Part model, mm, in its own coordinate system. Give positions to 0.01 mm unless a question says otherwise; leave off trailing zeros. Write each loop counter-clockwise with the first axis right and the second up, starting at its lowest first coordinate (ties: lowest second). Pieces come first, ordered by that corner, then holes. Notation, with made-up numbers: M 49,54 L 96,54 A16 cw 96,80 Z; hole C 22.5,8.5 d2. An arc over 180 degrees is marked long. Use a Markdown table: item, result.
```python
from build123d import *

# Parameters (mm, degrees)
SKETCH3_W                      = 333.036830712
SKETCH3_H                      = 85
BASE_FLANGE1_DEPTH             = 3
EDGE_FLANGE1_STRIP_W           = 13.4732
EDGE_FLANGE1_STRIP_H           = 3
EDGE_FLANGE1_STRIP_CUT_DEPTH   = 333.036830711
EDGE_FLANGE1_STRIP_2_W         = 13.4732
EDGE_FLANGE1_STRIP_2_H         = 3
EDGE_FLANGE1_STRIP_CUT_2_DEPTH = 333.036830711
EDGE_FLANGE1_DEPTH             = 333.036830711
EDGE_FLANGE1_BEND_DEPTH        = 333.036830711
SKETCH14_R                     = 4.1
CUT_EXTRUDE1_DEPTH             = 10
LPATTERN1_COUNT                = 3
LPATTERN1_PITCH                = 20
INDENT1_START                  = 23
INDENT1_DEPTH                  = 87
INDENT1_START_2                = 1066.181520764
INDENT1_2_DEPTH                = 11.708931468
INDENT1_START_3                = 23.50429019
INDENT1_3_DEPTH                = 85
INDENT1_START_4                = 1388.984464138
INDENT1_4_DEPTH                = 10.233887338
INDENT1_5_DEPTH                = 85
CUT_EXTRUDE2_DEPTH             = 10
LPATTERN2_COUNT                = 2
LPATTERN2_PITCH                = 101
LPATTERN2_COPY_1_SKETCH_R      = 4.1
LPATTERN2_COPY_1_DEPTH         = 10
LPATTERN2_COPY_2_SKETCH_R      = 4.1
LPATTERN2_COPY_2_DEPTH         = 10


with BuildPart() as part:
    # Base-Flange1: sheet metal written as solids
    # Sketch3 → Base-Flange1 (new body)
    with BuildSketch(Plane(origin=(-0.035963347, 187.801831242, 0), x_dir=(0.9999999816645936, 0.0001914962472965804, 0), z_dir=(-0.0001914962472965804, 0.9999999816645936, 0))):
        with Locations((1232.69993612, -66.00429019)):
            Rectangle(SKETCH3_W, SKETCH3_H)
    extrude(amount=-BASE_FLANGE1_DEPTH)

    # Edge-Flange1: sheet metal written as solids
    # Edge-Flange1 strip (on a plane across the edge) → Edge-Flange1 strip cut (cut)
    with BuildSketch(Plane(origin=(1399.182936963, 185.06977636, 108.50429019), x_dir=(0, 0, -1), z_dir=(-0.9999999816645935, -0.00019149624729661617, 0))):
        with Locations((-3, -1.5)):
            Rectangle(EDGE_FLANGE1_STRIP_W, EDGE_FLANGE1_STRIP_H)
    extrude(amount=EDGE_FLANGE1_STRIP_CUT_DEPTH, mode=Mode.SUBTRACT)

    # Edge-Flange1 strip 2 (on a plane across the edge) → Edge-Flange1 strip cut 2 (cut)
    with BuildSketch(Plane(origin=(1066.146112358, 185.006001057, 23.50429019), x_dir=(0, 0, 1), z_dir=(0.9999999816645935, 0.00019149624729661617, 0))):
        with Locations((-3, -1.5)):
            Rectangle(EDGE_FLANGE1_STRIP_2_W, EDGE_FLANGE1_STRIP_2_H)
    extrude(amount=EDGE_FLANGE1_STRIP_CUT_2_DEPTH, mode=Mode.SUBTRACT)

    # Edge-Flange1 section (on a plane across the edge) → Edge-Flange1 (add)
    with BuildSketch(Plane(origin=(1399.182936963, 185.06977636, 108.50429019), x_dir=(0, 0, -1), z_dir=(-0.9999999816645935, -0.00019149624729661617, 0))):
        with BuildLine():
            Line((0, 0.7366), (0, 12))
            Line((0, 12), (3, 12))
            Line((3, 12), (3, 0.7366))
            ThreePointArc((3, 0.7366), (3.215745145, 0.215745145), (3.7366, 0))
            Line((3.7366, 0), (3.7366, -3))
            ThreePointArc((3.7366, -3), (1.094424801, -1.905575199), (0, 0.7366))
        make_face()
    extrude(amount=EDGE_FLANGE1_DEPTH)

    # Edge-Flange1 section 2 (on a plane across the edge) → Edge-Flange1 bend (add)
    with BuildSketch(Plane(origin=(1066.146112358, 185.006001057, 23.50429019), x_dir=(0, 0, 1), z_dir=(0.9999999816645935, 0.00019149624729661617, 0))):
        with BuildLine():
            Line((0, 0.7366), (0, 12))
            Line((0, 12), (3, 12))
            Line((3, 12), (3, 0.7366))
            ThreePointArc((3, 0.7366), (3.215745145, 0.215745145), (3.7366, 0))
            Line((3.7366, 0), (3.7366, -3))
            ThreePointArc((3.7366, -3), (1.094424801, -1.905575199), (0, 0.7366))
        make_face()
    extrude(amount=EDGE_FLANGE1_BEND_DEPTH)

    # Sketch14 → Cut-Extrude1 (cut)
    with BuildSketch(Plane(origin=(-0.035963347, 187.801831242, 0), x_dir=(0.9999999816645936, 0.00019149624729658044, 0), z_dir=(-0.00019149624729658044, 0.9999999816645936, 0))):
        with Locations(Location((1152.844912527, -41.50429019, 0), (0, 0, 180))):
            Circle(SKETCH14_R)
        with Locations(Location((1213.814912527, -41.50429019, 0), (0, 0, 180))):
            Circle(SKETCH14_R)
        with Locations(Location((1152.844912527, -90.50429019, 0), (0, 0, 180))):
            Circle(SKETCH14_R)
        with Locations(Location((1213.814912527, -90.50429019, 0), (0, 0, 180))):
            Circle(SKETCH14_R)
    cut_extrude1 = extrude(amount=-CUT_EXTRUDE1_DEPTH, mode=Mode.SUBTRACT)

    # LPattern1: Cut-Extrude1 ×3
    with Locations(*[Vector(-0.9999999816645936, -0.00019149624729658041, 0) * (i * LPATTERN1_PITCH) for i in range(1, LPATTERN1_COUNT)]):
        add(cut_extrude1, mode=Mode.SUBTRACT)

    # Indent1: read off the stored shape, not the designer's step
    # Indent1 outline → Indent1 (cut)
    with BuildSketch(Plane.XY.offset(INDENT1_START)):
        with BuildLine():
            Line((1391.658769663, 190), (1390.104573792, 188.068047026))
            ThreePointArc((1390.104573792, 188.068047026), (1387.312839815, 180.67842019), (1389.429552771, 173.067908404))
            Line((1389.429552771, 173.067908404), (1390.14074534, 172))
            Line((1390.14074534, 172), (1399.185439777, 172))
            Line((1399.185439777, 172), (1401, 172))
            Line((1401, 172), (1401, 190))
            Line((1401, 190), (1391.658769663, 190))
        make_face()
        with BuildLine():
            Line((1076.353702039, 188.007964899), (1074.752112936, 190))
            Line((1074.752112936, 190), (1065, 190))
            Line((1065, 190), (1065, 172))
            Line((1065, 172), (1066.14860296, 172))
            Line((1066.14860296, 172), (1076.353013915, 172))
            Line((1076.353013915, 172), (1077.024720786, 173.00808405))
            ThreePointArc((1077.024720786, 173.00808405), (1079.143304168, 180.617808163), (1076.353702039, 188.007964899))
        make_face()
    extrude(amount=INDENT1_DEPTH, mode=Mode.SUBTRACT)

    # Sketch15 → Cut-Extrude2 (cut)
    with BuildSketch(Plane(origin=(-0.035963347, 187.801831242, 0), x_dir=(0.9999999816645936, 0.0001914962472966162, 0), z_dir=(-0.0001914962472966162, 0.9999999816645936, 0))):
        with BuildLine():
            Line((1290.140555319, -48.00429019), (1340.140555319, -48.00429019))
            ThreePointArc((1340.140555319, -48.00429019), (1358.140555319, -66.00429019), (1340.140555319, -84.00429019))
            Line((1340.140555319, -84.00429019), (1290.140555319, -84.00429019))
            ThreePointArc((1290.140555319, -84.00429019), (1272.140555319, -66.00429019), (1290.140555319, -48.00429019))
        make_face()
    extrude(amount=-CUT_EXTRUDE2_DEPTH, mode=Mode.SUBTRACT)

    # LPattern2: Cut-Extrude1 ×2
    with Locations(*[Vector(0.9999999816645935, 0.0001914962472965804, 0) * (i * LPATTERN2_PITCH) for i in range(1, LPATTERN2_COUNT)]):
        add(cut_extrude1, mode=Mode.SUBTRACT)

    # LPattern2 copy 1 sketch → LPattern2 copy 1 (cut)
    with BuildSketch(Plane(origin=(80.964035168, 187.817342438, 0), x_dir=(0.9999999816645936, 0.00019149624729658044, 0), z_dir=(-0.00019149624729658044, 0.9999999816645936, 0))):
        with Locations(Location((1152.844912527, -41.50429019, 0), (0, 0, 180))):
            Circle(LPATTERN2_COPY_1_SKETCH_R)
        with Locations(Location((1213.814912527, -41.50429019, 0), (0, 0, 180))):
            Circle(LPATTERN2_COPY_1_SKETCH_R)
        with Locations(Location((1152.844912527, -90.50429019, 0), (0, 0, 180))):
            Circle(LPATTERN2_COPY_1_SKETCH_R)
        with Locations(Location((1213.814912527, -90.50429019, 0), (0, 0, 180))):
            Circle(LPATTERN2_COPY_1_SKETCH_R)
    extrude(amount=-LPATTERN2_COPY_1_DEPTH, mode=Mode.SUBTRACT)

    # LPattern2 copy 2 sketch → LPattern2 copy 2 (cut)
    with BuildSketch(Plane(origin=(60.964035535, 187.813512513, 0), x_dir=(0.9999999816645936, 0.00019149624729658044, 0), z_dir=(-0.00019149624729658044, 0.9999999816645936, 0))):
        with Locations(Location((1152.844912527, -41.50429019, 0), (0, 0, 180))):
            Circle(LPATTERN2_COPY_2_SKETCH_R)
        with Locations(Location((1213.814912527, -41.50429019, 0), (0, 0, 180))):
            Circle(LPATTERN2_COPY_2_SKETCH_R)
        with Locations(Location((1152.844912527, -90.50429019, 0), (0, 0, 180))):
            Circle(LPATTERN2_COPY_2_SKETCH_R)
        with Locations(Location((1213.814912527, -90.50429019, 0), (0, 0, 180))):
            Circle(LPATTERN2_COPY_2_SKETCH_R)
    extrude(amount=-LPATTERN2_COPY_2_DEPTH, mode=Mode.SUBTRACT)


with BuildPart() as body_2:
    # Indent1 2 outline → Indent1 2 (new body)
    with BuildSketch(Plane(origin=(0, 0, 0), x_dir=(-0.00019149624731436396, 0.9999999816645935, 0), z_dir=(0.9999999816645936, 0.00019149624731436393, 0)).offset(INDENT1_START_2)):
        with BuildLine():
            ThreePointArc((184.801834685, 27.24089019), (184.58608954, 26.720035335), (184.065234685, 26.50429019))
            Line((184.065234685, 26.50429019), (172.801834685, 26.50429019))
            Line((172.801834685, 26.50429019), (172.801834685, 23.50429019))
            Line((172.801834685, 23.50429019), (184.065234685, 23.50429019))
            ThreePointArc((184.065234685, 23.50429019), (186.707409883, 24.598714992), (187.801834685, 27.24089019))
            Line((187.801834685, 27.24089019), (187.801834685, 104.76769019))
            ThreePointArc((187.801834685, 104.76769019), (186.707409884, 107.409865389), (184.065234685, 108.50429019))
            Line((184.065234685, 108.50429019), (172.801834685, 108.50429019))
            Line((172.801834685, 108.50429019), (172.801834685, 105.50429019))
            Line((172.801834685, 105.50429019), (184.065234685, 105.50429019))
            ThreePointArc((184.065234685, 105.50429019), (184.58608954, 105.288545045), (184.801834685, 104.76769019))
            Line((184.801834685, 104.76769019), (184.801834685, 27.24089019))
        make_face()
    extrude(amount=INDENT1_2_DEPTH)

    # Indent1 3 outline → Indent1 3 (cut)
    with BuildSketch(Plane.XY.offset(INDENT1_START_3)):
        with BuildLine():
            Line((1077.855992631, 180.052424815), (1077.854469122, 188.008243218))
            Line((1077.854469122, 188.008243218), (1074.619319449, 188.007634777))
            ThreePointArc((1074.619319449, 188.007634777), (1077.015456668, 184.346487369), (1077.855992631, 180.052424815))
        make_face()
        with BuildLine():
            ThreePointArc((1077.855992631, 180.052424815), (1077.230304306, 176.325431683), (1075.420572237, 173.007776861))
            Line((1075.420572237, 173.007776861), (1077.857341566, 173.008243493))
            Line((1077.857341566, 173.008243493), (1077.855992631, 180.052424815))
        make_face()
    extrude(amount=INDENT1_3_DEPTH, mode=Mode.SUBTRACT)


with BuildPart() as body_3:
    # Indent1 4 outline → Indent1 4 (new body)
    with BuildSketch(Plane(origin=(0, 0, 0), x_dir=(-0.00019149624729552394, 0.9999999816645935, 0), z_dir=(0.9999999816645936, 0.0001914962472955239, 0)).offset(INDENT1_START_4)):
        with BuildLine():
            ThreePointArc((187.801834685, 104.76769019), (186.707409884, 107.409865389), (184.065234685, 108.50429019))
            Line((184.065234685, 108.50429019), (172.801834685, 108.50429019))
            Line((172.801834685, 108.50429019), (172.801834685, 105.50429019))
            Line((172.801834685, 105.50429019), (184.065234685, 105.50429019))
            ThreePointArc((184.065234685, 105.50429019), (184.58608954, 105.288545045), (184.801834685, 104.76769019))
            Line((184.801834685, 104.76769019), (184.801834685, 27.24089019))
            ThreePointArc((184.801834685, 27.24089019), (184.58608954, 26.720035335), (184.065234685, 26.50429019))
            Line((184.065234685, 26.50429019), (172.801834685, 26.50429019))
            Line((172.801834685, 26.50429019), (172.801834685, 23.50429019))
            Line((172.801834685, 23.50429019), (184.065234685, 23.50429019))
            ThreePointArc((184.065234685, 23.50429019), (186.707409883, 24.598714992), (187.801834685, 27.24089019))
            Line((187.801834685, 27.24089019), (187.801834685, 104.76769019))
        make_face()
    extrude(amount=INDENT1_4_DEPTH)

    # Indent1 5 outline → Indent1 5 (cut)
    with BuildSketch(Plane.XY.offset(INDENT1_START_3)):
        with BuildLine():
            ThreePointArc((1391.482231002, 173.068301484), (1389.602669792, 176.366092083), (1388.950000203, 180.105369497))
            Line((1388.950000203, 180.105369497), (1388.951347768, 173.067816829))
            Line((1388.951347768, 173.067816829), (1391.482231002, 173.068301484))
        make_face()
        with BuildLine():
            Line((1392.336768964, 188.068477256), (1388.948475324, 188.067816554))
            Line((1388.948475324, 188.067816554), (1388.950000203, 180.105369497))
            ThreePointArc((1388.950000203, 180.105369497), (1389.831468968, 184.432237107), (1392.336768964, 188.068477256))
        make_face()
    extrude(amount=INDENT1_5_DEPTH, mode=Mode.SUBTRACT)


solid = part.part
```
1. Drop flat-ended pins along their axis: P1, Ø23.5, axis at x = 1248.5, z = 76.5, coming from the +Y side; P2, Ø10.5, axis at x = 1173.78, z = 41.5, coming from the -Y side; P3, Ø13, axis at x = 1314.78, z = 90.5, coming from the -Y side; P4, Ø6.5, axis at x = 1314.78, z = 41.5, coming from the +Y side. Give the stop position or say it passes through.
Findings below:
| item | result |
|---|---|
| P1 | y = 188.04 |
| P2 | y = 185.03 |
| P3 | y = 185.05 |
| P4 | through |
2. Cut at B-B, the plane z = 64. Give the cut face in (x, y), then the cut area to 3 significant figures.
Findings below:
| item | result |
|---|---|
| outline | M 1076.35,188.01 A12.7 cw 1078.15,185.01 L 1272.22,185.05 L 1272.22,188.05 Z; M 1357.99,185.06 L 1388.31,185.07 A12.7 cw 1390.1,188.07 L 1357.99,188.06 Z |
| area | 678 mm2 |
3. Drill centre lines: L1, parallel to Z at x = 1280, y = 183.5; L2, parallel to Y at x = 1178, z = 52; L3, parallel to Z at x = 1255, y = 187.25. Where is each one in solid material? Low to high.
Findings below:
| item | result |
|---|---|
| L1 | 23.5 to 26.5, 105.5 to 108.5 |
| L2 | 185.03 to 188.03 |
| L3 | 24.94 to 37.58, 45.43 to 86.58, 94.43 to 107.07 |
4. Cut at A-A, the plane y = 181. Give the cut face in (x, z).
Findings below:
| item | result |
|---|---|
| outline | M 1079.12,23.5 L 1387.33,23.5 L 1387.33,26.5 L 1079.12,26.5 Z; M 1079.12,105.5 L 1387.33,105.5 L 1387.33,108.5 L 1079.12,108.5 Z |
5. Two-plate mould, pull along X, no slides. Class faces 1 (the cylindrical face through (1076.56, 187.744, 65.806)), 2 (the cylindrical face through (1272.11, 186.57, 66.4)), 3 (the flat face through (1231, 179, 23.504)), 4 (the cylindrical face through (1128.9, 186.54, 42.74)): released by +X, released by -X, zero draft, split by the parting line, or undercut.
Findings below:
| item | result |
|---|---|
| face 1 | released by -X |
| face 2 | undercut |
| face 3 | zero draft |
| face 4 | undercut |
6. Cut at C-C, the plane z = 101. Give the cut face in (x, y).
Findings below:
| item | result |
|---|---|
| outline | M 1076.35,188.01 A12.7 cw 1078.15,185.01 L 1388.31,185.07 A12.7 cw 1390.1,188.07 Z |
